from build123d import *

# Parameters (mm, degrees)
F1_DEPTH     = 100
F3_DEPTH     = 3
F5_DEPTH     = 10
F6_R         = 1.5
F7_DEPTH     = 55.001
F8_T1_DEPTH  = 26.4990384046
F8_T3_DEPTH  = 43
F8_T5_DEPTH  = 64
F8_T7_DEPTH  = 26.4990384046
F8_T10_ANGLE = 90
F8_T12_ANGLE = 90
F8_T14_ANGLE = 90
F8_T16_ANGLE = 90
F9_W         = 5.2690437883
F9_H         = 22.4438142031
F10_DEPTH    = 25
F11_DEPTH    = 22.3
F12_R        = 5


# Not quite as in the source:
# - a fillet or chamfer that OpenCascade refuses, or shapes differently, is made with other operations: its cross-section is extruded or revolved along the edge and cut away or added
# - two fillets or chamfers of one size are made in one step


with BuildPart() as f1:
    # F0 (on Top) → F1 (new body)
    with BuildSketch(Plane.XY):
        with BuildLine():
            Line((-21.5, 35), (21.5, 35))
            ThreePointArc((21.5, 35), (23.6213203436, 34.1213203436), (24.5, 32))
            Line((24.5, 32), (24.5, 13.625))
            Line((24.5, 13.625), (30.5, 13.625))
            Line((30.5, 13.625), (30.5, 14.625))
            Line((30.5, 14.625), (28.5, 14.625))
            ThreePointArc((28.5, 14.625), (26.3786796564, 15.5036796564), (25.5, 17.625))
            Line((25.5, 17.625), (25.5, 32))
            ThreePointArc((25.5, 32), (24.3284271247, 34.8284271247), (21.5, 36))
            Line((21.5, 36), (-21.5, 36))
            ThreePointArc((-21.5, 36), (-24.3284271247, 34.8284271247), (-25.5, 32))
            Line((-25.5, 32), (-25.5, -32))
            ThreePointArc((-25.5, -32), (-24.3284271247, -34.8284271247), (-21.5, -36))
            Line((-21.5, -36), (21.5, -36))
            ThreePointArc((21.5, -36), (24.3284271247, -34.8284271247), (25.5, -32))
            Line((25.5, -32), (25.5, -17.625))
            ThreePointArc((25.5, -17.625), (26.3786796564, -15.5036796564), (28.5, -14.625))
            Line((28.5, -14.625), (30.5, -14.625))
            Line((30.5, -14.625), (30.5, -13.625))
            Line((30.5, -13.625), (24.5, -13.625))
            Line((24.5, -13.625), (24.5, -32))
            ThreePointArc((24.5, -32), (23.6213203436, -34.1213203436), (21.5, -35))
            Line((21.5, -35), (-21.5, -35))
            ThreePointArc((-21.5, -35), (-23.6213203436, -34.1213203436), (-24.5, -32))
            Line((-24.5, -32), (-24.5, 32))
            ThreePointArc((-24.5, 32), (-23.6213203436, 34.1213203436), (-21.5, 35))
        make_face()
    extrude(amount=F1_DEPTH)

    # F2 (on face) → F3 (join)
    with BuildSketch(Plane.XY.offset(100)):
        with BuildLine():
            Line((24.5, -32), (24.5, -13.625))
            Line((24.5, -13.625), (24.5, 0))
            Line((24.5, 0), (-24.5, 0))
            Line((-24.5, 0), (-24.5, -32))
            ThreePointArc((-24.5, -32), (-23.6213203436, -34.1213203436), (-21.5, -35))
            Line((-21.5, -35), (21.5, -35))
            ThreePointArc((21.5, -35), (23.6213203436, -34.1213203436), (24.5, -32))
        make_face()
        with BuildLine():
            Line((30.5, -13.625), (24.5, -13.625))
            Line((24.5, -13.625), (24.5, -32))
            ThreePointArc((24.5, -32), (23.6213203436, -34.1213203436), (21.5, -35))
            Line((21.5, -35), (-21.5, -35))
            ThreePointArc((-21.5, -35), (-23.6213203436, -34.1213203436), (-24.5, -32))
            Line((-24.5, -32), (-24.5, 0))
            Line((-24.5, 0), (-24.5, 30))
            Line((-24.5, 30), (-24.5, 32))
            ThreePointArc((-24.5, 32), (-23.6213203436, 34.1213203436), (-21.5, 35))
            Line((-21.5, 35), (21.5, 35))
            ThreePointArc((21.5, 35), (23.6213203436, 34.1213203436), (24.5, 32))
            Line((24.5, 32), (24.5, 30))
            Line((24.5, 30), (24.5, 13.625))
            Line((24.5, 13.625), (30.5, 13.625))
            Line((30.5, 13.625), (30.5, 14.625))
            Line((30.5, 14.625), (28.5, 14.625))
            ThreePointArc((28.5, 14.625), (26.3786796564, 15.5036796564), (25.5, 17.625))
            Line((25.5, 17.625), (25.5, 32))
            ThreePointArc((25.5, 32), (24.3284271247, 34.8284271247), (21.5, 36))
            Line((21.5, 36), (-21.5, 36))
            ThreePointArc((-21.5, 36), (-24.3284271247, 34.8284271247), (-25.5, 32))
            Line((-25.5, 32), (-25.5, -32))
            ThreePointArc((-25.5, -32), (-24.3284271247, -34.8284271247), (-21.5, -36))
            Line((-21.5, -36), (21.5, -36))
            ThreePointArc((21.5, -36), (24.3284271247, -34.8284271247), (25.5, -32))
            Line((25.5, -32), (25.5, -17.625))
            ThreePointArc((25.5, -17.625), (26.3786796564, -15.5036796564), (28.5, -14.625))
            Line((28.5, -14.625), (30.5, -14.625))
            Line((30.5, -14.625), (30.5, -13.625))
        make_face()
        with BuildLine():
            Line((-24.5, 32), (-24.5, 30))
            Line((-24.5, 30), (24.5, 30))
            Line((24.5, 30), (24.5, 32))
            ThreePointArc((24.5, 32), (23.6213203436, 34.1213203436), (21.5, 35))
            Line((21.5, 35), (-21.5, 35))
            ThreePointArc((-21.5, 35), (-23.6213203436, 34.1213203436), (-24.5, 32))
        make_face()
    extrude(amount=F3_DEPTH)

    # F4 (on face) → F5 (join, symmetric)
    with BuildSketch(Plane(origin=(0, 0, 0), x_dir=(1, 0, 0), z_dir=(0, 0, -1))):
        with BuildLine():
            Line((23.3, -13.625), (23.3, -32))
            ThreePointArc((23.3, -32), (22.7727922061, -33.2727922061), (21.5, -33.8))
            Line((21.5, -33.8), (-21.5, -33.8))
            ThreePointArc((-21.5, -33.8), (-22.7727922061, -33.2727922061), (-23.3, -32))
            Line((-23.3, -32), (-23.3, 32))
            ThreePointArc((-23.3, 32), (-22.7727922061, 33.2727922061), (-21.5, 33.8))
            Line((-21.5, 33.8), (21.5, 33.8))
            ThreePointArc((21.5, 33.8), (22.7727922061, 33.2727922061), (23.3, 32))
            Line((23.3, 32), (23.3, 13.625))
            Line((23.3, 13.625), (24.5, 13.625))
            Line((24.5, 13.625), (24.5, 32))
            ThreePointArc((24.5, 32), (23.6213203436, 34.1213203436), (21.5, 35))
            Line((21.5, 35), (-21.5, 35))
            ThreePointArc((-21.5, 35), (-23.6213203436, 34.1213203436), (-24.5, 32))
            Line((-24.5, 32), (-24.5, -32))
            ThreePointArc((-24.5, -32), (-23.6213203436, -34.1213203436), (-21.5, -35))
            Line((-21.5, -35), (21.5, -35))
            ThreePointArc((21.5, -35), (23.6213203436, -34.1213203436), (24.5, -32))
            Line((24.5, -32), (24.5, -13.625))
            Line((24.5, -13.625), (23.3, -13.625))
        make_face()
    extrude(amount=F5_DEPTH, both=True)

    # F6 (on face) → F7 (cut, through all)
    with BuildSketch(Plane(origin=(-24.5, 0, 0), x_dir=(0, -1, 0), z_dir=(-1, 0, 0))):
        with Locations((-20, -5)):
            Circle(F6_R)
        with Locations((20, -5)):
            Circle(F6_R)
    extrude(amount=-F7_DEPTH, mode=Mode.SUBTRACT)

    # F8: fillet of radius 5 on 1 edges, made by hand

    # F8_s2 → F8_t1 (cut)
    with BuildSketch(Plane.XZ.offset(-32)):
        with BuildLine():
            ThreePointArc((24.5, 10), (23.6095842402, 8.4824354457), (23.3, 6.7503846381))
            Line((23.3, 6.7503846381), (23.3, 10))
            Line((23.3, 10), (24.5, 10))
        make_face()
    extrude(amount=F8_T1_DEPTH, mode=Mode.SUBTRACT)

    # F8_s4 → F8_t3 (cut)
    with BuildSketch(Plane.YZ.offset(-21.5)):
        with BuildLine():
            ThreePointArc((35, 10), (34.1095842402, 8.4824354457), (33.8, 6.7503846381))
            Line((33.8, 6.7503846381), (33.8, 10))
            Line((33.8, 10), (35, 10))
        make_face()
        with BuildLine():
            ThreePointArc((-35, 10), (-34.1095842402, 8.4824354457), (-33.8, 6.7503846381))
            Line((-33.8, 6.7503846381), (-33.8, 10))
            Line((-33.8, 10), (-35, 10))
        make_face()
    extrude(amount=F8_T3_DEPTH, mode=Mode.SUBTRACT)

    # F8_s6 → F8_t5 (cut)
    with BuildSketch(Plane.XZ.offset(-32)):
        with BuildLine():
            ThreePointArc((-24.5, 10), (-23.6095842402, 8.4824354457), (-23.3, 6.7503846381))
            Line((-23.3, 6.7503846381), (-23.3, 10))
            Line((-23.3, 10), (-24.5, 10))
        make_face()
    extrude(amount=F8_T5_DEPTH, mode=Mode.SUBTRACT)

    # F8_s8 → F8_t7 (cut)
    with BuildSketch(Plane.XZ.offset(5.5009615954)):
        with BuildLine():
            ThreePointArc((24.5, 10), (23.6095842402, 8.4824354457), (23.3, 6.7503846381))
            Line((23.3, 6.7503846381), (23.3, 10))
            Line((23.3, 10), (24.5, 10))
        make_face()
    extrude(amount=F8_T7_DEPTH, mode=Mode.SUBTRACT)

    # F8_s9 → F8_t10 (revolve, cut)
    with BuildSketch(Plane.XZ.offset(-32)):
        with BuildLine():
            ThreePointArc((24.5, 10), (23.6095842402, 8.4824354457), (23.3, 6.7503846381))
            Line((23.3, 6.7503846381), (23.3, 10))
            Line((23.3, 10), (24.5, 10))
        make_face()
    revolve(axis=Axis((21.5, 32, 10), (0, 0, 1)), revolution_arc=F8_T10_ANGLE, mode=Mode.SUBTRACT)

    # F8_s11 → F8_t12 (revolve, cut)
    with BuildSketch(Plane.YZ.offset(-21.5)):
        with BuildLine():
            ThreePointArc((35, 10), (34.1095842402, 8.4824354457), (33.8, 6.7503846381))
            Line((33.8, 6.7503846381), (33.8, 10))
            Line((33.8, 10), (35, 10))
        make_face()
    revolve(axis=Axis((-21.5, 32, 10), (0, 0, 1)), revolution_arc=F8_T12_ANGLE, mode=Mode.SUBTRACT)

    # F8_s13 → F8_t14 (revolve, cut)
    with BuildSketch(Plane.XZ.offset(32)):
        with BuildLine():
            ThreePointArc((-24.5, 10), (-23.6095842402, 8.4824354457), (-23.3, 6.7503846381))
            Line((-23.3, 6.7503846381), (-23.3, 10))
            Line((-23.3, 10), (-24.5, 10))
        make_face()
    revolve(axis=Axis((-21.5, -32, 10), (0, 0, 1)), revolution_arc=F8_T14_ANGLE, mode=Mode.SUBTRACT)

    # F8_s15 → F8_t16 (revolve, cut)
    with BuildSketch(Plane.YZ.offset(21.5)):
        with BuildLine():
            ThreePointArc((-35, 10), (-34.1095842402, 8.4824354457), (-33.8, 6.7503846381))
            Line((-33.8, 6.7503846381), (-33.8, 10))
            Line((-33.8, 10), (-35, 10))
        make_face()
    revolve(axis=Axis((21.5, -32, 10), (0, 0, 1)), revolution_arc=F8_T16_ANGLE, mode=Mode.SUBTRACT)

    # F9 (on face) → F10 (cut)
    with BuildSketch(Plane.XY.offset(103)):
        with Locations((21.8654781058, -11.2219071016)):
            Rectangle(F9_W, F9_H)
    extrude(amount=-F10_DEPTH, mode=Mode.SUBTRACT)

    # F9 (on face) → F11 (cut)
    with BuildSketch(Plane.XY.offset(103)):
        Polygon((24.5, -13.625), (24.5, 0), (19.2309562117, 0), (19.2309562117, -22.4438142031), (24.5, -22.4438142031), align=None)
    extrude(amount=-F11_DEPTH, mode=Mode.SUBTRACT)

    # F12
    f12_edges = [f1.edges().sort_by_distance(p)[0] for p in [
        (-24.5, 0, 101.5),
        (19.230956, 0, 101.5),
        (-24.5, 30, 101.5),
        (24.5, 30, 101.5),
    ]]
    fillet(f12_edges, radius=F12_R)


solid = f1.part
Verification items for the finished model (mm, model axes). A direction names the side the tool comes from. Give positions to 0.01 mm unless a question says otherwise; leave off trailing zeros. Write each loop counter-clockwise with the first axis right and the second up, starting at its lowest first coordinate (ties: lowest second). Pieces come first, ordered by that corner, then holes. Notation, with made-up numbers: (12.5, 24.5) - (64.5, 24.5) arc R25 ccw to (64.5, 63.5) - close; hole circle Ø8 at (81, -16). An arc over 180 degrees is marked (long way). Answer as CSV lines item,"result". Start each with the question number.
1. Sectioned sample at A-A (y = 20). Record the boundary of the cut face in (x, z), then the cut area to 3 significant figures.
2. Thickness scan on line 1 (Y direction, x = 3, z = 56); line 2 (X direction, y = 25, z = 13); line 3 (Z direction, x = -4.5, y = -19.5). Record the ranges inside material, lowest first.
3. Sectioned sample at B-B (x = -12.5). Record the boundary of the cut face in (y, z).
4. Set-up check for faces 1 (the face through (-23.6, -34.14, 54.37)), 2 (the face through (23.3, -23, -2)), 3 (the face through (24.5, -23, -5)), 4 (the face through (-23, 28.57, 101.52)), 5 (the face through (-23.64, 34.1, -5.07)): record each of +Z, -Z, +X, -X, +Y, -Y from which the full face is reachable in a straight line by a thin tool's end or side.
5. Sectioned sample at D-D (y = -20). Record the boundary of the cut face in (x, z).
6. Draft check along Y on faces 6 (the face through (0, 35, 54)), 7 (the face through (0, 35, -5)), 8 (the face through (-25, 0, 0)), 9 (the face through (23.62, -22.68, 8.51)). Enter one of: pulls with the +Y half, pulls with the -Y half, needs draft (parallel to the pull), parting line crosses it, or undercut.
7. Sectioned sample at C-C (z = 3.5). Record the boundary of the cut face in (x, y) (3 decimals).
8. Depth check by flat-ended pin: pin 1 (7 mm diameter, centred on y = 22, z = 34.5, fed in from +X); pin 2 (8 mm diameter, centred on y = 6, z = -5.5, fed in from -X); pin 3 (11 mm diameter, centred on y = -24.5, z = -6.5, fed in from +X). Enter the tip coordinate at first touch or a pass-through.
Derived:
1,outline,"(-25.5, 0) - (-24.5, 0) - (-24.5, -3.5) - (-23.3, -3.5) - (-23.3, 6.75) arc R5 ccw to (-24.5, 10) - (-24.5, 103) - (-25.5, 103) - close; (-24.5, -10) - (-23.3, -10) - (-23.3, -6.5) - (-24.5, -6.5) - close; (23.3, -10) - (24.5, -10) - (24.5, -6.5) - (23.3, -6.5) - close; (23.3, -3.5) - (24.5, -3.5) - (24.5, 0) - (25.5, 0) - (25.5, 103) - (24.5, 103) - (24.5, 10) arc R5 ccw to (23.3, 6.75) - close"
1,area,"244 mm²"
2,line 1,"-36 to -35, 35 to 36"
2,line 2,"-25.5 to -24.5, 24.5 to 25.5"
2,line 3,"100 to 103"
3,outline,"(-36, 0) - (-35, 0) - (-35, -10) - (-33.8, -10) - (-33.8, 6.75) arc R5 ccw to (-35, 10) - (-35, 100) - (0, 100) - (0, 103) - (-36, 103) - close; (30, 100) - (35, 100) - (35, 10) arc R5 ccw to (33.8, 6.75) - (33.8, -10) - (35, -10) - (35, 0) - (36, 0) - (36, 103) - (30, 103) - close"
4,face 1,"none"
4,face 2,"-Z"
4,face 3,"-Z, +X, +Y, -Y"
4,face 4,"+Z"
4,face 5,"-Z, -X, +Y"
5,outline,"(-25.5, 0) - (-24.5, 0) - (-24.5, -3.5) - (-23.3, -3.5) - (-23.3, 6.75) arc R5 ccw to (-24.5, 10) - (-24.5, 100) - (19.23, 100) - (19.23, 103) - (-25.5, 103) - close; (-24.5, -10) - (-23.3, -10) - (-23.3, -6.5) - (-24.5, -6.5) - close; (23.3, -10) - (24.5, -10) - (24.5, -6.5) - (23.3, -6.5) - close; (23.3, -3.5) - (24.5, -3.5) - (24.5, 0) - (25.5, 0) - (25.5, 103) - (24.5, 103) - (24.5, 10) arc R5 ccw to (23.3, 6.75) - close"
6,face 6,"undercut"
6,face 7,"pulls with the +Y half"
6,face 8,"needs draft"
6,face 9,"undercut"
7,outline,"(-25.5, -32) arc R4 ccw to (-21.5, -36) - (21.5, -36) arc R4 ccw to (25.5, -32) - (25.5, -17.625) arc R3 cw to (28.5, -14.625) - (30.5, -14.625) - (30.5, -13.625) - (23.3, -13.625) - (23.3, -32) arc R1.8 cw to (21.5, -33.8) - (-21.5, -33.8) arc R1.8 cw to (-23.3, -32) - (-23.3, 32) arc R1.8 cw to (-21.5, 33.8) - (21.5, 33.8) arc R1.8 cw to (23.3, 32) - (23.3, 13.625) - (30.5, 13.625) - (30.5, 14.625) - (28.5, 14.625) arc R3 cw to (25.5, 17.625) - (25.5, 32) arc R4 ccw to (21.5, 36) - (-21.5, 36) arc R4 ccw to (-25.5, 32) - close"
8,pin 1,"x = 25.5"
8,pin 2,"x = -24.5"
8,pin 3,"x = 24.5"
